Source: CAD feature listing. Evaluate the final solid. Frame: model axes, mm. A direction names the side the tool comes from. Round coordinates to 2 decimals unless told otherwise and drop trailing zeros. Loops run counter-clockwise (first coordinate to the right, second up) from the corner with the lowest first, then second, coordinate; pieces in that order, holes last.
(1) Set-up query: faces 4 (the flat face through (22, 0, -15)), 5 (the flat face through (11.507, -0.448, -9.33)), 6 (the cylindrical face through (-29, -28, 3)). Return all of +Z, -Z, +X, -X, +Y, -Y with unobstructed straight access to the full face (end or side cutting, diameter ignored); none if empty.
(2) Mould query, pull axis Y, two halves, no side actions, for faces 1 (the flat face through (0, 32, 10)), 2 (the cylindrical face through (25.9, 27.86, -12.04)), 3 (the flat face through (-22, 0, -15)). Classes: pulls with the +Y half, pulls with the -Y half, needs draft (parallel to the pull), parting line crosses it, or undercut.
(3) Section C-C, the plane y = 3.5. Return the cut outline in (x, z), plus the area to 3 significant figures.
(4) Section A-A, the plane z = 0.25. Return the cut outline in (x, y).
(5) First-contact query: pin 1 Ø9 at (x, y) = (-25, 25) entering from +Z. Flat tip, straight axial feed; report the tip coordinate or a pass-through.
(6) Section B-B, the plane z = 12.75. Return the cut outline in (x, y), plus the area to 3 significant figures.
(7) Section D-D, the plane z = -6.5. Return the cut outline in (x, y).
(8) Material intervals for probe 1 along Y at (x, z) = (25, -10.45); probe 2 along Y at (x, z) = (25, 3.25); probe 3 along X at (y, z) = (18, 2), sorted ascending.
```python
from build123d import *

# Parameters (mm, degrees)
F1_DEPTH = 15
F3_DEPTH = 64
F4_R     = 5
F4_R_2   = 3
F5_DEPTH = 24


with BuildPart() as f1:
    # F0 (on Top) → F1 (new body, symmetric)
    with BuildSketch(Plane.XY):
        with BuildLine():
            Line((25, -32), (32, -32))
            Line((32, -32), (32, -25))
            Line((32, -25), (28, -25))
            ThreePointArc((28, -25), (27.1213203436, -27.1213203436), (25, -28))
            Line((25, -28), (25, -32))
        make_face()
        with BuildLine():
            Line((12, -32), (25, -32))
            Line((25, -32), (25, -28))
            ThreePointArc((25, -28), (22.8786796564, -22.8786796564), (28, -25))
            Line((28, -25), (32, -25))
            Line((32, -25), (32, 25))
            Line((32, 25), (28, 25))
            ThreePointArc((28, 25), (22.8786796564, 22.8786796564), (25, 28))
            Line((25, 28), (25, 32))
            Line((25, 32), (-25, 32))
            Line((-25, 32), (-25, 28))
            ThreePointArc((-25, 28), (-22.8786796564, 27.1213203436), (-22, 25))
            ThreePointArc((-22, 25), (-25, 22), (-28, 25))
            Line((-28, 25), (-32, 25))
            Line((-32, 25), (-32, -25))
            Line((-32, -25), (-28, -25))
            ThreePointArc((-28, -25), (-25, -22), (-22, -25))
            ThreePointArc((-22, -25), (-22.8786796564, -27.1213203436), (-25, -28))
            Line((-25, -28), (-25, -32))
            Line((-25, -32), (-12, -32))
            Line((-12, -32), (12, -32))
        make_face()
        with BuildLine():
            Line((28, 25), (32, 25))
            Line((32, 25), (32, 32))
            Line((32, 32), (25, 32))
            Line((25, 32), (25, 28))
            ThreePointArc((25, 28), (27.1213203436, 27.1213203436), (28, 25))
        make_face()
        with BuildLine():
            Line((-32, -32), (-25, -32))
            Line((-25, -32), (-25, -28))
            ThreePointArc((-25, -28), (-27.1213203436, -27.1213203436), (-28, -25))
            Line((-28, -25), (-32, -25))
            Line((-32, -25), (-32, -32))
        make_face()
        with BuildLine():
            Line((-25, 28), (-25, 32))
            Line((-25, 32), (-32, 32))
            Line((-32, 32), (-32, 25))
            Line((-32, 25), (-28, 25))
            ThreePointArc((-28, 25), (-27.1213203436, 27.1213203436), (-25, 28))
        make_face()
        with BuildLine():
            Line((12, -32), (25, -32))
            Line((25, -32), (25, -28))
            ThreePointArc((25, -28), (22.8786796564, -22.8786796564), (28, -25))
            Line((28, -25), (32, -25))
            Line((32, -25), (32, 25))
            Line((32, 25), (28, 25))
            ThreePointArc((28, 25), (22.8786796564, 22.8786796564), (25, 28))
            Line((25, 28), (25, 32))
            Line((25, 32), (-25, 32))
            Line((-25, 32), (-25, 28))
            ThreePointArc((-25, 28), (-22.8786796564, 27.1213203436), (-22, 25))
            ThreePointArc((-22, 25), (-25, 22), (-28, 25))
            Line((-28, 25), (-32, 25))
            Line((-32, 25), (-32, -25))
            Line((-32, -25), (-28, -25))
            ThreePointArc((-28, -25), (-25, -22), (-22, -25))
            ThreePointArc((-22, -25), (-22.8786796564, -27.1213203436), (-25, -28))
            Line((-25, -28), (-25, -32))
            Line((-25, -32), (-12, -32))
            Line((-12, -32), (12, -32))
        make_face()
    extrude(amount=F1_DEPTH, both=True)

    # F2 (on face) → F3 (cut)
    with BuildSketch(Plane.XZ.offset(32)):
        with BuildLine():
            Line((-11, -3.5), (-12, -15))
            Line((-12, -15), (0, -15))
            Line((0, -15), (0, -14.5))
            ThreePointArc((0, -14.5), (-7.7781745931, -11.2781745931), (-11, -3.5))
        make_face()
        with BuildLine():
            Line((0, -3.5), (-11, -3.5))
            ThreePointArc((-11, -3.5), (-7.7781745931, -11.2781745931), (0, -14.5))
            Line((0, -14.5), (0, -3.5))
        make_face()
        with BuildLine():
            Line((0, -3.5), (0, -14.5))
            ThreePointArc((0, -14.5), (7.7781745931, -11.2781745931), (11, -3.5))
            Line((11, -3.5), (0, -3.5))
        make_face()
        with BuildLine():
            Line((0, -14.5), (0, -15))
            Line((0, -15), (12, -15))
            Line((12, -15), (11, -3.5))
            ThreePointArc((11, -3.5), (7.7781745931, -11.2781745931), (0, -14.5))
        make_face()
        with BuildLine():
            ThreePointArc((11, -3.5), (7.7781745931, 4.2781745931), (0, 7.5))
            Line((0, 7.5), (0, -3.5))
            Line((0, -3.5), (11, -3.5))
        make_face()
        with BuildLine():
            ThreePointArc((0, 7.5), (-7.7781745931, 4.2781745931), (-11, -3.5))
            Line((-11, -3.5), (0, -3.5))
            Line((0, -3.5), (0, 7.5))
        make_face()
    extrude(amount=-F3_DEPTH, mode=Mode.SUBTRACT)

    # F4 (on face) → F5 (cut)
    with BuildSketch(Plane.XY.offset(15)):
        with Locations((-25, -25)):
            Circle(F4_R)
        with Locations((-25, -25)):
            Circle(F4_R_2, mode=Mode.SUBTRACT)
        with Locations((-25, 25)):
            Circle(F4_R)
        with Locations((-25, 25)):
            Circle(F4_R_2, mode=Mode.SUBTRACT)
        with Locations((25, 25)):
            Circle(F4_R)
        with Locations((25, 25)):
            Circle(F4_R_2, mode=Mode.SUBTRACT)
        with Locations((25, -25)):
            Circle(F4_R)
        with Locations((25, -25)):
            Circle(F4_R_2, mode=Mode.SUBTRACT)
        with Locations((-25, -25)):
            Circle(F4_R_2)
        with Locations((25, -25)):
            Circle(F4_R_2)
        with Locations((25, 25)):
            Circle(F4_R_2)
        with Locations((-25, 25)):
            Circle(F4_R_2)
    extrude(amount=-F5_DEPTH, mode=Mode.SUBTRACT)


solid = f1.part
```
Output values:
1. face 4: -Z, +X, -X, +Y, -Y
1. face 5: -Z, +Y, -Y
1. face 6: +Z
2. face 1: pulls with the +Y half
2. face 2: undercut
2. face 3: needs draft
3. outline: (-32, -15) - (-12, -15) - (-11, -3.5) arc R11 cw to (11, -3.5) - (12, -15) - (32, -15) - (32, 15) - (-32, 15) - close
3. area: 1,470 mm2
4. outline: (-32, -32) - (-10.34, -32) - (-10.34, 32) - (-32, 32) - close; (10.34, -32) - (32, -32) - (32, 32) - (10.34, 32) - close; hole circle Ø10 at (-25, -25); hole circle Ø10 at (-25, 25); hole circle Ø10 at (25, -25); hole circle Ø10 at (25, 25)
5. pin 1: stops at z = -9
6. outline: (-32, -32) - (32, -32) - (32, 32) - (-32, 32) - close; hole circle Ø10 at (-25, -25); hole circle Ø10 at (-25, 25); hole circle Ø10 at (25, -25); hole circle Ø10 at (25, 25)
6. area: 3,780 mm2
7. outline: (-32, -32) - (-11.26, -32) - (-11.26, 32) - (-32, 32) - close; (11.26, -32) - (32, -32) - (32, 32) - (11.26, 32) - close; hole circle Ø10 at (-25, -25); hole circle Ø10 at (-25, 25); hole circle Ø10 at (25, -25); hole circle Ø10 at (25, 25)
8. probe 1: y = -32 to -28, -22 to 22, 28 to 32
8. probe 2: y = -32 to -30, -20 to 20, 30 to 32
8. probe 3: x = -32 to -9.53, 9.53 to 32
